Source: CAD feature listing. Evaluate the final solid. Frame: model axes, mm. Face numbers are marked on the shaded views. Give positions to 0.01 mm unless a question says otherwise; leave off trailing zeros. Order: outer loops, then holes, each group sorted by start corner. A loop starts at its lowest first (then second) coordinate and runs counter-clockwise, first axis right, second up. Notation, with made-up numbers: M 61,69.5 L 82,69.5 A30 cw 82,106.5 Z; hole C 32.5,47.25 d3. An arc over 180 degrees is marked long. Answer as a JSON object with one key per item and string values. Group by question number.
1. Section query A-A (z = 0). Output: boundary loops of the cut face in (x, y), plus the area to 3 significant figures.
2. Material intervals for L1, parallel to Y at x = 10.5, z = -32; L2, parallel to X at y = 25, z = 0, sorted ascending. Write a range as [from, to].
3. Pin query (flat end, axial travel): P1, Ø5, axis at y = 20.5, z = -16, coming from the +X side; P2, Ø6, axis at x = -6, y = 26.5, coming from the +Z side; P3, Ø1.5, axis at y = 13, z = -10.5, coming from the +X side; P4, Ø23, axis at x = 0, z = 0, coming from the +Y side. Return the tip coordinate at first contact, or that it passes through.
4. Section query B-B (x = 0). Output: boundary loops of the cut face in (y, z).
5. Pull-direction query (Y, two-part tool) for the marked faces 1, 2, 3 and 4; classes: +Y half, -Y half, draft (parallel to the pull), parting line (faces both ways), or undercut.
6. Section query D-D (x = 21). Output: boundary loops of the cut face in (y, z), plus the area to 3 significant figures.
7. Section query C-C (y = 14). Output: boundary loops of the cut face in (x, z).
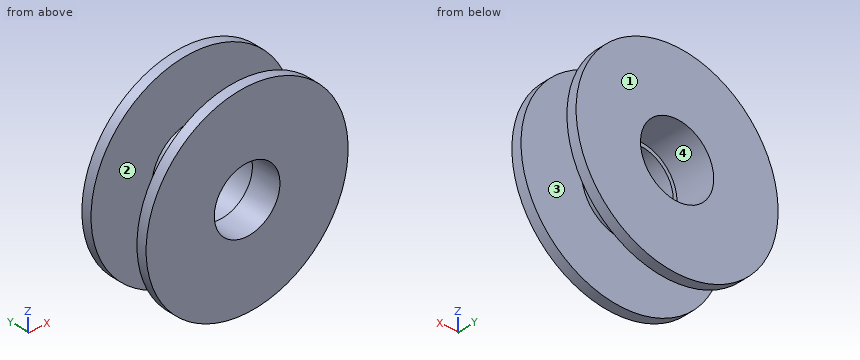
from build123d import *

# Parameters (mm, degrees)
CUT_EXTRUDE1_START = 48
SKETCH2_R          = 14.5
CUT_EXTRUDE1_DEPTH = 48


with BuildPart() as part:
    # Sketch1 → Revolve1 (revolve)
    with BuildSketch(Plane(origin=(0, 0, 0), x_dir=(0, 0, -1), z_dir=(1, 0, 0))):
        Polygon((-16, 9.838658872), (-40, 9.838658872), (-40, 5.838658872), (-13, 5.838658872), (-13, 17.838658872), (-14.5, 17.838658872), (-14.5, 29.838658872), (-16, 29.838658872), align=None)
    revolve1 = revolve(axis=Axis((0, 28.058626224, 0), (0, -1, 0)))

    # Mirror3: Revolve1 across plane
    add(revolve1.mirror(Plane.ZX.offset(19.838658872)))

    # Sketch2 → Cut-Extrude1 (cut)
    with BuildSketch(Plane(origin=(0, 17.838658872, 0), x_dir=(1, 0, 0), z_dir=(0, 1, 0)).offset(CUT_EXTRUDE1_START)):
        with Locations(Location((0, 0, 0), (0, 0, 270))):
            Circle(SKETCH2_R)
    extrude(amount=-CUT_EXTRUDE1_DEPTH, mode=Mode.SUBTRACT)


solid = part.part
Answer sheet:
{
 "1": {"outline": "M -40,5.84 L -13,5.84 L -13,17.84 L -14.5,17.84 L -14.5,33.84 L -40,33.84 L -40,29.84 L -16,29.84 L -16,9.84 L -40,9.84 Z; M 13,5.84 L 40,5.84 L 40,9.84 L 16,9.84 L 16,29.84 L 40,29.84 L 40,33.84 L 14.5,33.84 L 14.5,17.84 L 13,17.84 Z", "area": "504 mm^2"},
 "2": {"L1": "[5.84, 9.84], [29.84, 33.84]", "L2": "[-16, -14.5], [14.5, 16]"},
 "3": {"P1": "x = 8.59", "P2": "z = 15.72", "P3": "x = 12.69", "P4": "through"},
 "4": {"outline": "M 5.84,-40 L 9.84,-40 L 9.84,-16 L 29.84,-16 L 29.84,-40 L 33.84,-40 L 33.84,-14.5 L 17.84,-14.5 L 17.84,-13 L 5.84,-13 Z; M 5.84,13 L 17.84,13 L 17.84,14.5 L 33.84,14.5 L 33.84,40 L 29.84,40 L 29.84,16 L 9.84,16 L 9.84,40 L 5.84,40 Z"},
 "5": {"face 1": "+Y half", "face 2": "undercut", "face 3": "undercut", "face 4": "draft"},
 "6": {"outline": "M 5.84,-34.04 L 9.84,-34.04 L 9.84,34.04 L 5.84,34.04 Z; M 29.84,-34.04 L 33.84,-34.04 L 33.84,34.04 L 29.84,34.04 Z", "area": "545 mm^2"},
 "7": {"outline": "C 0,0 d32; hole C 0,0 d26"}
}
